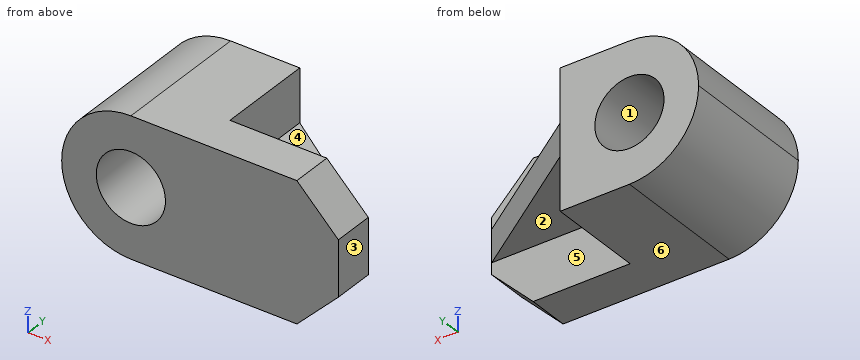
```python
from build123d import *

# Parameters (mm, degrees)
BOSS_EXTRUDE2_DEPTH      = 381
BOSS_EXTRUDE2_DEPTH_BACK = 381
FILLET1_R                = 381
SKETCH2_W                = 762
SKETCH2_H                = 292.1
CUT_EXTRUDE1_DEPTH       = 533.4
SKETCH4_R                = 190.5
CUT_EXTRUDE2_DEPTH       = 1746.961339778
CHAMFER1_SIZE            = 228.6


with BuildPart() as part:
    # Sketch1 → Boss-Extrude2 (new, two sides: drawn at the far end of the back side and taken through both)
    with BuildSketch(Plane.XY.offset(-BOSS_EXTRUDE2_DEPTH_BACK)):
        Polygon((0, 0), (0, 762), (762, 762), (1524, 228.6), (1524, 0), align=None)
    extrude(amount=BOSS_EXTRUDE2_DEPTH + BOSS_EXTRUDE2_DEPTH_BACK)

    # Fillet1
    fillet1_edges = [part.edges().sort_by_distance(p)[0] for p in [
        (0, 381, -381),
        (0, 381, 381),
    ]]
    fillet(fillet1_edges, radius=FILLET1_R - 0.0001)  # a hair under: the kernel refuses the full size

    # Sketch2 → Cut-Extrude1 (cut)
    with BuildSketch(Plane(origin=(0, 762, 0), x_dir=(1, 0, 0), z_dir=(0, 1, 0))):
        with Locations((1143, 234.95)):
            Rectangle(SKETCH2_W, SKETCH2_H)
        with Locations((1143, -234.95)):
            Rectangle(SKETCH2_W, SKETCH2_H)
    extrude(amount=-CUT_EXTRUDE1_DEPTH, mode=Mode.SUBTRACT)

    # Sketch4 → Cut-Extrude2 (cut, through all)
    with BuildSketch(Plane(origin=(0, 762, 0), x_dir=(1, 0, 0), z_dir=(0, 1, 0))):
        with Locations(Location((381, 0, 0), (0, 0, 270))):
            Circle(SKETCH4_R)
    extrude(amount=-CUT_EXTRUDE2_DEPTH, mode=Mode.SUBTRACT)

    # Chamfer1
    chamfer1_edges = [part.edges().sort_by_distance(p)[0] for p in [
        (1524, 114.3, 381),
        (1524, 114.3, -381),
    ]]
    chamfer(chamfer1_edges, length=CHAMFER1_SIZE)


solid = part.part
```
CAD build for the part. Positions are in the model's coordinates, mm. Face numbers are marked on the shaded views. A direction names the side the tool comes from. Coordinates: 2 decimals unless noted, no trailing zeros. Write each loop counter-clockwise with the first axis right and the second up, starting at its lowest first coordinate (ties: lowest second). Pieces come first, ordered by that corner, then holes. Notation, with made-up numbers: (67.5, 21) -> (103.5, 21) arc R19 ccw to (103.5, 39) -> close; hole circle Ø4 at (18.25, 52). An arc over 180 degrees is marked (long way). Return JSON: item names as keys, results as strings. Group by question number.
Q1. Cut at D-D, the plane x = 339. Give the cut face in (y, z).
Q2. Pull direction X, two halves, no side cores. Call the marked faces 1, 2 and 3: released by +X, released by -X, zero draft, split by the parting line, or undercut.
Q3. Which spindle directions (+Z, -Z, +X, -X, +Y, -Y) get a long thin tool onto all of the face, cutting with end or side? Do the marked faces 4, 5 and 6. Say none if no direction does.
Q4. Cut at B-B, the plane x = 1205. Give the cut face in (y, z), then the cut area to 3 significant figures.
Q5. Flat gauge pins, fed straight in: pin 1 (3 mm diameter, centred on y = 341.5, z = -65, fed in from +X); pin 2 (3 mm diameter, centred on x = 295, y = 662.5, fed in from +Z); pin 3 (4 mm diameter, centred on y = 612, z = -92, fed in from +X). Where does each tip first touch, or does it go through?
Q6. Cut at A-A, the plane z = 19. Give the cut face in (x, y).
Q7. Drill centre lines: line 1 (X direction, y = 175, z = 0); line 2 (Z direction, x = 295, y = 115.5); line 3 (Y direction, x = 1005.5, z = -301.5). Where is each one in solid material? Low to high.
Returned:
{
 "1": {"outline": "(0, -378.68) -> (762, -378.68) -> (762, -185.81) -> (0, -185.81) -> close; (0, 185.81) -> (762, 185.81) -> (762, 378.68) -> (0, 378.68) -> close"},
 "2": {"face 1": "undercut", "face 2": "zero draft", "face 3": "released by +X"},
 "3": {"face 4": "+Z, +X, +Y", "face 5": "-Z, +X, +Y", "face 6": "-Z, +X, -X, +Y, -Y"},
 "4": {"outline": "(0, -381) -> (228.6, -381) -> (228.6, -88.9) -> (451.9, -88.9) -> (451.9, 88.9) -> (228.6, 88.9) -> (228.6, 381) -> (0, 381) -> close", "area": "214,000 mm2"},
 "5": {"pin 1": "stops at x = 1364.86", "pin 2": "stops at z = 371.51", "pin 3": "stops at x = 762"},
 "6": {"outline": "(0.47, 0) -> (191.45, 0) -> (191.45, 762) -> (0.47, 762) -> close; (570.55, 0) -> (1524, 0) -> (1524, 228.6) -> (762, 762) -> (570.55, 762) -> close"},
 "7": {"line 1": "x = 0 to 190.5, 571.5 to 1524", "line 2": "z = -371.17 to -169.98, 169.98 to 371.17", "line 3": "y = 0 to 228.6"}
}
